Build history of the part. All positions in model axes, mm. A direction names the side the tool comes from. Round coordinates to 2 decimals unless told otherwise and drop trailing zeros. Write each loop counter-clockwise with the first axis right and the second up, starting at its lowest first coordinate (ties: lowest second). Pieces come first, ordered by that corner, then holes. Notation, with made-up numbers: (-16.5, -20.5) -> (25.5, -20.5) arc R20 cw to (25.5, 3.5) -> close; hole circle Ø11 at (82, 8). An arc over 180 degrees is marked (long way). Answer in a Markdown table with one row per item. Add a question column.
from build123d import *

# Parameters (mm, degrees)
F0_W     = 900
F0_H     = 2600
F1_DEPTH = 25
F3_DEPTH = 20


with BuildPart() as f1:
    # F0 (on Front) → F1 (new body)
    with BuildSketch(Plane.XZ):
        Rectangle(F0_W, F0_H)
    extrude(amount=F1_DEPTH)

    # F2 (on face) → F3 (cut)
    with BuildSketch(Plane.XZ.offset(25)):
        with BuildLine():
            Line((250, -600), (250, 900))
            ThreePointArc((250, 900), (0, 1150), (-250, 900))
            Line((-250, 900), (-250, -600))
            ThreePointArc((-250, -600), (0, -850), (250, -600))
        make_face()
        with BuildLine():
            ThreePointArc((-210, 900), (0, 1110), (210, 900))
            Line((210, 900), (210, -600))
            ThreePointArc((210, -600), (0, -810), (-210, -600))
            Line((-210, -600), (-210, 900))
        make_face(mode=Mode.SUBTRACT)
    extrude(amount=-F3_DEPTH, mode=Mode.SUBTRACT)


solid = f1.part
(1) Saw through at C-C (x = 0). List the corners of the cut face in (y, z), plus the area to 3 significant figures.
(2) Saw through at A-A (y = -18.75). List the corners of the cut face in (x, z), plus the area to 3 significant figures.
(3) Mould opens along Z. For faces 1 (the face through (221, -5, 155)), 2 (the face through (-3, -25, 163)) say: pulls with the +Z half, pulls with the -Z half, needs draft (parallel to the pull), parting line crosses it, or undercut.
(4) Which spindle directions (+Z, -Z, +X, -X, +Y, -Y) get a long thin tool onto all of the face, cutting with end or side? Do faces 3 (the face through (5.5, -15.14, 1149.94)), 4 (the face through (-306, -25, 18)). Say none if no direction does.
(5) Probe line 1 along X through (y, z) = (-12.25, 865); line 2 along X through (y, z) = (-15, 1093.5); line 3 along Z through (x, y) = (-54.5, -14). List the from-to ranges inside material, lowest first.
(6) Saw through at B-B (z = 301.5). List the corners of the cut face in (x, y), plus the area to 3 significant figures.
Answer sheet:
| question | item | result |
|---|---|---|
| 1 | outline | (-25, -1300) -> (0, -1300) -> (0, 1300) -> (-25, 1300) -> (-25, 1150) -> (-5, 1150) -> (-5, 1110) -> (-25, 1110) -> (-25, -810) -> (-5, -810) -> (-5, -850) -> (-25, -850) -> close |
| 1 | area | 63,400 mm² |
| 2 | outline | (-450, -1300) -> (450, -1300) -> (450, 1300) -> (-450, 1300) -> close; (-210, -600) arc R210 ccw to (210, -600) -> (210, 900) arc R210 ccw to (-210, 900) -> close; hole (-250, -600) arc R250 ccw to (250, -600) -> (250, 900) arc R250 ccw to (-250, 900) -> close |
| 2 | area | 2,160,000 mm² |
| 3 | face 1 | undercut |
| 3 | face 2 | needs draft |
| 4 | face 3 | -Y |
| 4 | face 4 | +Z, -Z, +X, -X, -Y |
| 5 | line 1 | x = -450 to -250, -210 to 210, 250 to 450 |
| 5 | line 2 | x = -450 to -158.3, -81.6 to 81.6, 158.3 to 450 |
| 5 | line 3 | z = -1300 to -843.99, -802.8 to 1102.8, 1143.99 to 1300 |
| 6 | outline | (-450, -25) -> (-250, -25) -> (-250, -5) -> (-210, -5) -> (-210, -25) -> (210, -25) -> (210, -5) -> (250, -5) -> (250, -25) -> (450, -25) -> (450, 0) -> (-450, 0) -> close |
| 6 | area | 20,900 mm² |
